Input: part model. Units: mm. Frame: model coordinates. Face numbers are marked on the shaded views. A direction names the side the tool comes from. Coordinates: 2 decimals unless noted, no trailing zeros. Loops run counter-clockwise (first coordinate to the right, second up) from the corner with the lowest first, then second, coordinate; pieces in that order, holes last. Notation, with made-up numbers: M 10,7 L 21,7 A19 cw 21,30 Z; hole C 76.5,30.25 d4. An arc over 180 degrees is marked long. Use a Markdown table: item, result. Add a question column.
1. Section C-C on y = -8. Output: boundary loops of the cut face in (x, z).
2. Line query: L1, parallel to Y at x = 5.5, z = 20.5; L2, parallel to Z at x = 8, y = -2.5; L3, parallel to X at y = 11.5, z = 44. Output: solid intervals per line, ascending. Write a range as [from, to].
3. Section D-D on z = 28.5. Output: boundary loops of the cut face in (x, y), then the cut area to 3 significant figures.
4. Section A-A on x = 8. Output: boundary loops of the cut face in (y, z), then the cut area to 3 significant figures.
5. Draft query along Y for the marked faces 1, 2, 3 and 4. Return one class per face: +Y half, -Y half, draft (parallel to the pull), parting line (faces both ways), or undercut.
6. Section B-B on z = 23. Output: boundary loops of the cut face in (x, y).
7. Pin query (flat end, axial travel): pin 1 (1.7 mm diameter, centred on x = -5.66, y = 5.84, fed in from +Z); pin 2 (12 mm diameter, centred on x = 17, z = 35.5, fed in from +Y); pin 3 (4 mm diameter, centred on y = 16.5, z = 13, fed in from +X); pin 4 (16 mm diameter, centred on x = -8, z = 9, fed in from +Y). Return the tip coordinate at first contact, or that it passes through.
8. Set-up query: the marked faces 5, 6, 7 and 8. Return all of +Z, -Z, +X, -X, +Y, -Y with unobstructed straight access to the full face (end or side cutting, diameter ignored); none if empty.
```python
from build123d import *

# Parameters (mm, degrees)
PAD_DEPTH       = 50
POCKET_DEPTH    = 25
SKETCH002_R     = 2.6
POCKET001_DEPTH = 35.001
SKETCH003_R     = 5
POCKET002_DEPTH = 30
SKETCH004_R     = 5.2
SKETCH004_R_2   = 1.4
POCKET003_DEPTH = 25.001
CHAMFER_SIZE    = 1.5
CHAMFER001_SIZE = 1


with BuildPart() as part:
    # Sketch → Pad (new body)
    with BuildSketch(Plane.XY):
        with BuildLine():
            ThreePointArc((-33.433034, 10.5), (-18.5, 11.5), (-33.433034, 12.5))
            Line((-37.456439, 12.5), (-33.433034, 12.5))
            ThreePointArc((-26, 23), (-33.770135, 19.977912), (-37.456439, 12.5))
            Line((-26, 23), (26, 23))
            ThreePointArc((37.456439, 12.5), (33.770135, 19.977912), (26, 23))
            Line((33.433034, 12.5), (37.456439, 12.5))
            ThreePointArc((33.433034, 12.5), (18.5, 11.5), (33.433034, 10.5))
            Line((33.433034, 10.5), (37.456439, 10.5))
            ThreePointArc((32.598736, 2.081577), (35.960662, 5.752374), (37.456439, 10.5))
            Line((12.5, -12), (32.598736, 2.081577))
            Line((4, -12), (12.5, -12))
            Line((0, -14), (4, -12))
            Line((-4, -12), (0, -14))
            Line((-12.5, -12), (-4, -12))
            Line((-32.598736, 2.081577), (-12.5, -12))
            ThreePointArc((-37.456439, 10.5), (-35.960662, 5.752374), (-32.598736, 2.081577))
            Line((-37.456439, 10.5), (-33.433034, 10.5))
        make_face()
    extrude(amount=PAD_DEPTH)

    # Sketch001 (on Face19 of Pad) → Pocket (cut)
    with BuildSketch(Plane.XY.offset(50)):
        with BuildLine():
            Line((-26, 23), (26, 23))
            ThreePointArc((26, 23), (17.868272, 19.631728), (14.5, 11.5))
            Line((14.5, 3), (14.5, 11.5))
            ThreePointArc((11.5, 0), (13.62132, 0.87868), (14.5, 3))
            Line((-11.5, 0), (11.5, 0))
            ThreePointArc((-14.5, 3), (-13.62132, 0.87868), (-11.5, 0))
            Line((-14.5, 11.5), (-14.5, 3))
            ThreePointArc((-14.5, 11.5), (-17.868272, 19.631728), (-26, 23))
        make_face()
    extrude(amount=-POCKET_DEPTH, mode=Mode.SUBTRACT)

    # Sketch002 (on Face19 of Pocket) → Pocket001 (cut, through all)
    with BuildSketch(Plane.XZ.offset(12)):
        with Locations((-8, 41)):
            Circle(SKETCH002_R)
        with Locations((8, 41)):
            Circle(SKETCH002_R)
        with Locations((-8, 9)):
            Circle(SKETCH002_R)
        with Locations((8, 9)):
            Circle(SKETCH002_R)
    extrude(amount=-POCKET001_DEPTH, mode=Mode.SUBTRACT)

    # Sketch003 (on Face9 of Pocket001) → Pocket002 (cut)
    with BuildSketch(Plane(origin=(0, 23, 0), x_dir=(-1, 0, 0), z_dir=(0, 1, 0))):
        with Locations((-8, 41)):
            Circle(SKETCH003_R)
        with Locations((8, 41)):
            Circle(SKETCH003_R)
        with Locations((8, 9)):
            Circle(SKETCH003_R)
        with Locations((-8, 9)):
            Circle(SKETCH003_R)
    extrude(amount=-POCKET002_DEPTH, mode=Mode.SUBTRACT)

    # Sketch004 (on Face27 of Pocket002) → Pocket003 (cut, through all)
    with BuildSketch(Plane.XY.offset(25)):
        with Locations((0, 11.5)):
            Circle(SKETCH004_R)
        with Locations((-5.656854, 17.156854)):
            Circle(SKETCH004_R_2)
        with Locations((5.656854, 17.156854)):
            Circle(SKETCH004_R_2)
        with Locations((5.656854, 5.843146)):
            Circle(SKETCH004_R_2)
        with Locations((-5.656854, 5.843146)):
            Circle(SKETCH004_R_2)
    extrude(amount=-POCKET003_DEPTH, mode=Mode.SUBTRACT)

    # Chamfer
    chamfer_edges = [part.edges().sort_by_distance(p)[0] for p in [
        (17.868272, 19.631728, 50),
        (33.770135, 19.977912, 50),
        (14.5, 7.25, 50),
        (13.62132, 0.87868, 50),
        (0, 0, 50),
        (-13.62132, 0.87868, 50),
        (-14.5, 7.25, 50),
        (-17.868272, 19.631728, 50),
        (-33.770135, 19.977912, 50),
        (-35.960662, 5.752374, 50),
        (-22.549368, -4.959211, 50),
        (22.549368, -4.959211, 50),
        (35.960662, 5.752374, 50),
        (18.5, 11.5, 50),
        (-18.5, 11.5, 50),
        (33.770135, 19.977912, 0),
        (0, 23, 0),
        (-33.770135, 19.977912, 0),
        (-18.5, 11.5, 0),
        (-35.960662, 5.752374, 0),
        (-22.549368, -4.959211, 0),
        (22.549368, -4.959211, 0),
        (35.960662, 5.752374, 0),
        (18.5, 11.5, 0),
    ]]
    chamfer(chamfer_edges, length=CHAMFER_SIZE)

    # Chamfer001
    chamfer001_edges = [part.edges().sort_by_distance(p)[0] for p in [
        (-5.2, 11.5, 25),
    ]]
    chamfer(chamfer001_edges, length=CHAMFER001_SIZE)


solid = part.part
```
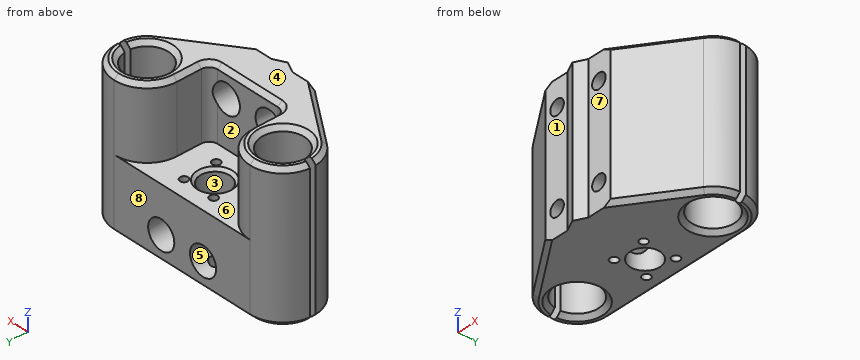
Answers below:
| question | item | result |
|---|---|---|
| 1 | outline | M -18.21,1.5 L -15.6,0 L 15.6,0 L 18.21,1.5 L 18.21,48.5 L 15.6,50 L -15.6,50 L -18.21,48.5 Z; hole C -8,9 d5.2; hole C -8,41 d5.2; hole C 8,9 d5.2; hole C 8,41 d5.2 |
| 2 | L1 | y = [-12, 4.45], [7.23, 15.77], [18.55, 23] |
| 2 | L2 | z = [0, 4], [14, 36], [46, 50] |
| 2 | L3 | x = [-18.5, -14.5], [14.5, 18.5] |
| 3 | outline | M -37.46,10.5 A11.5 ccw -32.6,2.08 L -12.5,-12 L -4,-12 L 0,-14 L 4,-12 L 12.5,-12 L 32.6,2.08 A11.5 ccw 37.46,10.5 L 33.43,10.5 A7.5 cw long 33.43,12.5 L 37.46,12.5 A11.5 ccw 14.5,11.5 L 14.5,3 A3 cw 11.5,0 L -11.5,0 A3 cw -14.5,3 L -14.5,11.5 A11.5 ccw -37.46,12.5 L -33.43,12.5 A7.5 cw long -33.43,10.5 Z |
| 3 | area | 1,040 mm² |
| 4 | outline | M -12,0 L 21.5,0 L 23,1.5 L 23,4 L -7,4 L -7,6.4 L -12,6.4 Z; M -12,11.6 L -7,11.6 L -7,14 L 23,14 L 23,25 L 0,25 L 0,36 L -7,36 L -7,38.4 L -12,38.4 Z; M -12,43.6 L -7,43.6 L -7,46 L 0,46 L 0,48.5 L -1.5,50 L -12,50 Z |
| 4 | area | 751 mm² |
| 5 | face 1 | -Y half |
| 5 | face 2 | +Y half |
| 5 | face 3 | undercut |
| 5 | face 4 | draft |
| 6 | outline | M -37.46,10.5 A11.5 ccw -32.6,2.08 L -12.5,-12 L -4,-12 L 0,-14 L 4,-12 L 12.5,-12 L 32.6,2.08 A11.5 ccw 37.46,10.5 L 33.43,10.5 A7.5 cw long 33.43,12.5 L 37.46,12.5 A11.5 ccw 26,23 L -26,23 A11.5 ccw -37.46,12.5 L -33.43,12.5 A7.5 cw long -33.43,10.5 Z; hole C -5.66,5.84 d2.8; hole C -5.66,17.16 d2.8; hole C 0,11.5 d10.4; hole C 5.66,5.84 d2.8; hole C 5.66,17.16 d2.8 |
| 7 | pin 1 | passes through |
| 7 | pin 2 | stops at y = 22.6 |
| 7 | pin 3 | stops at x = 37.1 |
| 7 | pin 4 | stops at y = 23 |
| 8 | face 5 | +Y |
| 8 | face 6 | +Z, +Y |
| 8 | face 7 | +Z, -Z, +X, -Y |
| 8 | face 8 | +Z, -Z, +X, -X, +Y |
